```python
from build123d import *

# Parameters (mm, degrees)
F0_W     = 304.8
F0_H     = 304.8
F1_DEPTH = 25.4
F2_W     = 7.9375
F2_H     = 304.8
F3_DEPTH = 158.75
F4_R     = 38.1
F5_DEPTH = 12.7
F6_R     = 9.525
F7_DEPTH = 12.7


with BuildPart() as f1:
    # F0 (on Right) → F1 (new body)
    with BuildSketch(Plane.YZ):
        Rectangle(F0_W, F0_H)
    extrude(amount=F1_DEPTH)

    # F2 (on face) → F3 (join)
    with BuildSketch(Plane.YZ.offset(25.4)):
        with Locations((148.43125, 0)):
            Rectangle(F2_W, F2_H)
    extrude(amount=F3_DEPTH)

    # F4 (on face) → F5 (join)
    with BuildSketch(Plane.YZ.offset(25.4)):
        Circle(F4_R)
    extrude(amount=F5_DEPTH)

    # F6 (on face) → F7 (cut)
    with BuildSketch(Plane.YZ.offset(25.4)):
        Circle(F6_R)
    extrude(amount=F7_DEPTH, mode=Mode.SUBTRACT)


solid = f1.part
```
The model under review builds one solid part; all positions refer to its coordinate system, in mm. A direction names the side the tool comes from. Round coordinates to 2 decimals unless told otherwise and drop trailing zeros. Write each loop counter-clockwise with the first axis right and the second up, starting at its lowest first coordinate (ties: lowest second). Pieces come first, ordered by that corner, then holes. Notation, with made-up numbers: (42.5, 54) -> (70.5, 54) arc R12 cw to (70.5, 65) -> close; hole circle Ø2 at (60.25, 3). An arc over 180 degrees is marked (long way). Use CSV: the item, a comma, the result in double quotes.
Q1. For pin 1 Ø1.5 at (y, z) = (-90.5, 7.5) entering from +X; pin 2 Ø4 at (x, z) = (160, 111.5) entering from -Y; pin 3 Ø6 at (x, y) = (36, 43.5) entering from -Z; pin 4 Ø15 at (y, z) = (0, 0) entering from -X, all flat-tipped, find the tip position at first contact; note any pin that passes through.
Checks:
pin 1,"x = 25.4"
pin 2,"y = 144.46"
pin 3,"through"
pin 4,"x = 0"
Q2. To check wall thickness, follow probe 1 along Z at (x, y) = (34.5, 0) (3 decimals); probe 2 along X at (y, z) = (4.5, -44); probe 3 along Y at (x, z) = (119.5, 32). State the ranges of each line that lie inside material, in increasing order. Write a range as [from, to].
Checks:
probe 1,"[-38.1, -9.525], [9.525, 38.1]"
probe 2,"[0, 25.4]"
probe 3,"[144.46, 152.4]"
Q3. Consider section B-B (y = 0). Give the boundary of the cut face in (x, z) (3 decimals), then the cut area to 3 significant figures.
Checks:
outline,"(0, -152.4) -> (25.4, -152.4) -> (25.4, -38.1) -> (38.1, -38.1) -> (38.1, -9.525) -> (25.4, -9.525) -> (25.4, 9.525) -> (38.1, 9.525) -> (38.1, 38.1) -> (25.4, 38.1) -> (25.4, 152.4) -> (0, 152.4) -> close"
area,"8,470 mm²"
Q4. Mouldability with a two-part tool opening along Z and no side actions: class faces 1 (the flat face through (38.1, 8, -8)), 2 (the flat face through (23, 33, 152.4)), 3 (the cylindrical face through (31.661, -7.559, -5.796)) as released by +Z, released by -Z, zero draft, split by the parting line, or undercut.
Checks:
face 1,"zero draft"
face 2,"released by +Z"
face 3,"undercut"
Q5. Consider section D-D (x = 54.5). Give the boundary of the cut face in (y, z), then the cut area to 3 significant figures.
Checks:
outline,"(144.46, -152.4) -> (152.4, -152.4) -> (152.4, 152.4) -> (144.46, 152.4) -> close"
area,"2,420 mm²"
Q6. For faces 4 (the flat face through (91, 152.4, -2)), 5 (the cylindrical face through (31.661, -30.235, -23.183)), list the 3-axis set-ups (+Z, -Z, +X, -X, +Y, -Y) from which the entire face can be reached by the end or side of a thin tool; tool diameter is ignored.
Checks:
face 4,"+Z, -Z, +X, -X, +Y"
face 5,"+X"
Q7. Consider section C-C (z = -77.5). Give the boundary of the cut face in (x, y), then the cut area to 3 significant figures.
Checks:
outline,"(0, -152.4) -> (25.4, -152.4) -> (25.4, 144.46) -> (184.15, 144.46) -> (184.15, 152.4) -> (0, 152.4) -> close"
area,"9,000 mm²"
